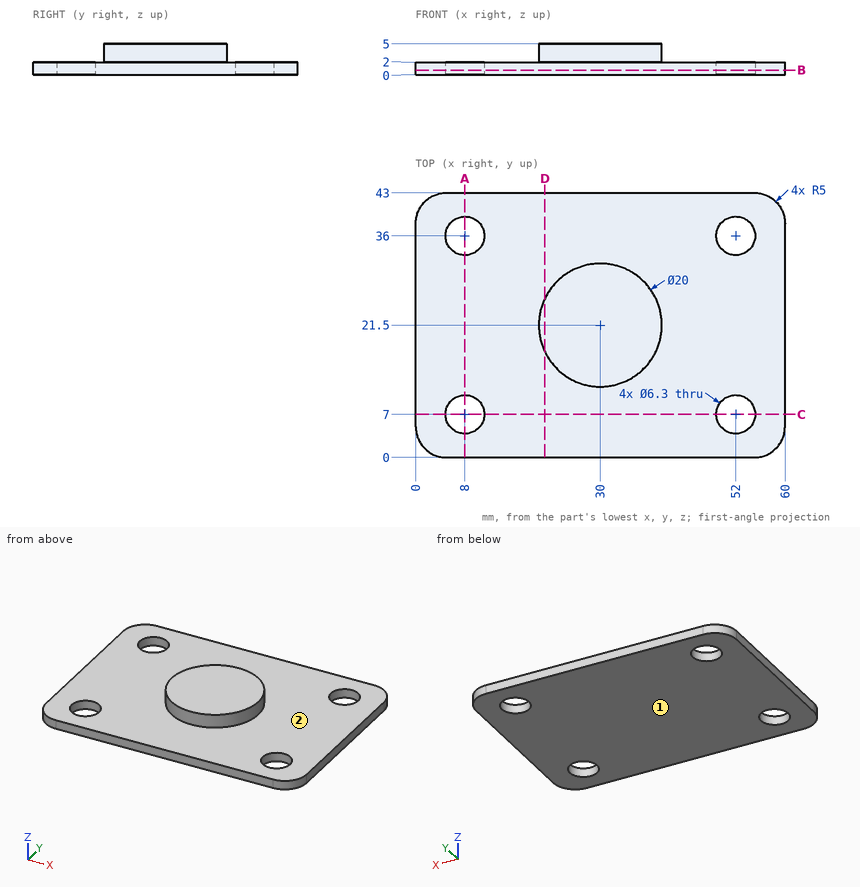
The drawing under review shows one solid part. Ordinate dimensions are in mm from its lowest x, y, z. A direction names the side the tool comes from. Round coordinates to 2 decimals unless told otherwise and drop trailing zeros. Write each loop counter-clockwise with the first axis right and the second up, starting at its lowest first coordinate (ties: lowest second). Pieces come first, ordered by that corner, then holes. Notation, with made-up numbers: (-14, 69.5) - (7, 69.5) arc R15 ccw to (7, 93.5) - close; hole circle Ø9 at (86, -21). An arc over 180 degrees is marked (long way). Put each result on its own line as item: value.
Q1. We need section C-C (y = 7). Give the boundary of the cut face in (x, z), and give its area (3 significant figures).
Solved:
outline: (0, 0) - (4.85, 0) - (4.85, 2) - (0, 2) - close; (11.15, 0) - (48.85, 0) - (48.85, 2) - (11.15, 2) - close; (55.15, 0) - (60, 0) - (60, 2) - (55.15, 2) - close
area: 94.8 mm2
Q2. We need section D-D (x = 21). Give the boundary of the cut face in (y, z).
Solved:
outline: (0, 0) - (43, 0) - (43, 2) - (25.86, 2) - (25.86, 5) - (17.14, 5) - (17.14, 2) - (0, 2) - close
Q3. We need section B-B (z = 0.75). Give the boundary of the cut face in (x, y), and give its area (3 significant figures).
Solved:
outline: (0, 5) arc R5 ccw to (5, 0) - (55, 0) arc R5 ccw to (60, 5) - (60, 38) arc R5 ccw to (55, 43) - (5, 43) arc R5 ccw to (0, 38) - close; hole circle Ø6.3 at (8, 7); hole circle Ø6.3 at (8, 36); hole circle Ø6.3 at (52, 7); hole circle Ø6.3 at (52, 36)
area: 2,430 mm2
Q4. We need section A-A (x = 8). Give the boundary of the cut face in (y, z).
Solved:
outline: (0, 0) - (3.85, 0) - (3.85, 2) - (0, 2) - close; (10.15, 0) - (32.85, 0) - (32.85, 2) - (10.15, 2) - close; (39.15, 0) - (43, 0) - (43, 2) - (39.15, 2) - close
Q5. Wall thickness on probe 1 along Y at (x, z) = (8, 1.35); probe 2 along Z at (x, y) = (50.5, 12.5); probe 3 along Y at (x, z) = (49.5, 1.85): over which ranges is each line inside the solid? List them lowest first.
Solved:
probe 1: y = 0 to 3.85, 10.15 to 32.85, 39.15 to 43
probe 2: z = 0 to 2
probe 3: y = 0 to 5.08, 8.92 to 34.08, 37.92 to 43
Q6. Machinability: for the marked faces 1 and 2, which of the approach directions +Z, -Z, +X, -X, +Y, -Y give a long, thin tool a straight path to every point of the face, cutting with its end or side? Answer none if there is none.
Solved:
face 1: -Z, +X, -X, +Y, -Y
face 2: +Z
Q7. Insertion check: pin 1 Ø8 at (x, y) = (8, 7) entering from +Z; pin 2 Ø1 at (y, z) = (26, 3) entering from -X; pin 3 Ø4 at (x, y) = (52, 7) entering from +Z. Each pin has a flat end and moves straight along its axis. Give the tip position at first contact, or say it passes through.
Solved:
pin 1: stops at z = 2
pin 2: stops at x = 20.83
pin 3: passes through
